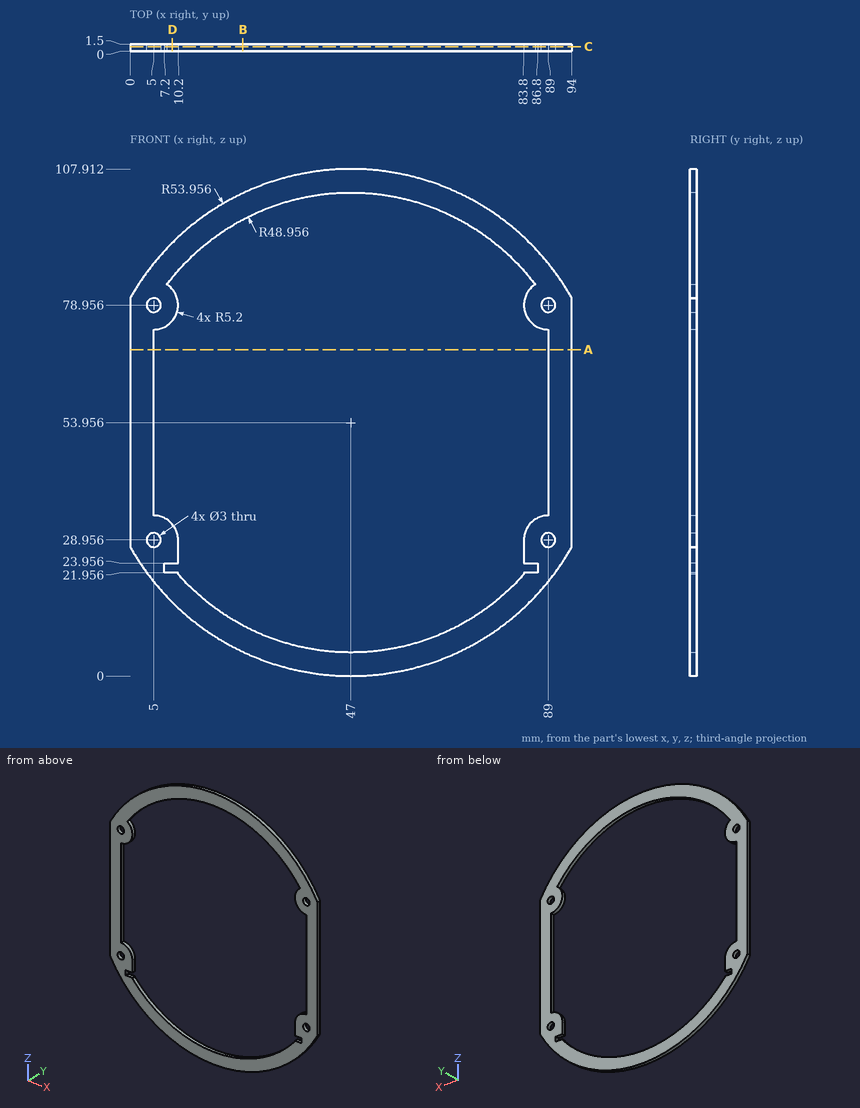
Can you work these out from the drawing? Everything is in mm from the part's minimum corner. Give positions to 0.01 mm unless a question says otherwise; leave off trailing zeros. Loops run counter-clockwise (first coordinate to the right, second up) from the corner with the lowest first, then second, coordinate; pieces in that order, holes last. Notation, with made-up numbers: (19.5, -37.5) -> (63.5, -37.5) arc R18 ccw to (63.5, -10.5) -> close; hole circle Ø2 at (-8.75, -25.75). An arc over 180 degrees is marked (long way). Write item = value, one per line.
1) Suppose I cut it at B-B on x = 24. Write out the boundary of the cut face in (y, z).
Check result:
outline = (0, 5.15) -> (1.5, 5.15) -> (1.5, 10.74) -> (0, 10.74) -> close; (0, 97.17) -> (1.5, 97.17) -> (1.5, 102.76) -> (0, 102.76) -> close
2) Will these pins go through, and if not, where does the flat tip stop? pin 1 (1.8 mm diameter, centred on x = 5, z = 78.956, fed in from -Y); pin 2 (0.8 mm diameter, centred on x = 8.5, y = 0.5, fed in from +Z).
Check result:
pin_1 = through
pin_2 = 92.16
3) I need wall thicknesses on L1, parallel to X at y = 0.2, z = 29; L2, parallel to X at y = 0.4, z = 54; L3, parallel to Z at x = 88.5, y = 0.4. Which ranges of each line are inside material? Lowest first, please. Write a range as from..to.
Check result:
L1 = 0..3.5, 6.5..10.2, 83.8..87.5, 90.5..94
L2 = 0..5, 89..94
L3 = 19.47..27.54, 30.37..34.13, 73.78..77.54, 80.37..88.44
4) Suppose I cut it at C-C on y = 0.95. Give the number of separate pieces and of enclosed holes in the cut face, then the cut area to 3 significant figures.
Check result:
separate_pieces = 1
enclosed_holes = 5
area = 1,710 mm2
5) Suppose I cut it at D-D on x = 9. Write out the boundary of the cut face in (y, z).
Check result:
outline = (0, 15.65) -> (1.5, 15.65) -> (1.5, 21.96) -> (0, 21.96) -> close; (0, 23.96) -> (1.5, 23.96) -> (1.5, 32.28) -> (0, 32.28) -> close; (0, 75.63) -> (1.5, 75.63) -> (1.5, 82.28) -> (0, 82.28) -> close; (0, 84.82) -> (1.5, 84.82) -> (1.5, 92.26) -> (0, 92.26) -> close
6) Suppose I cut it at A-A on z = 69.5. Write out the boundary of the cut face in (x, y).
Check result:
outline = (0, 0) -> (5, 0) -> (5, 1.5) -> (0, 1.5) -> close; (89, 0) -> (94, 0) -> (94, 1.5) -> (89, 1.5) -> close
